Source: CAD feature listing. Evaluate the final solid. Frame: model axes, mm. A direction names the side the tool comes from. Give positions to 0.01 mm unless a question says otherwise; leave off trailing zeros. Loops run counter-clockwise (first coordinate to the right, second up) from the corner with the lowest first, then second, coordinate; pieces in that order, holes last.
from build123d import *

# Parameters (mm, degrees)
F0_W      = 79
F0_H      = 58
F0_W_2    = 69
F0_H_2    = 46
F1_DEPTH  = 2
F2_W      = 15
F2_H      = 5
F3_DEPTH  = 10
F5_DEPTH  = 20
F6_W      = 75
F6_H      = 20
F7_DEPTH  = 5
F8_R      = 1
F9_DEPTH  = 5
F10_R     = 1
F11_DEPTH = 79.001
F12_W     = 5
F12_H     = 2
F13_DEPTH = 69
F14_ANGLE = 180


with BuildPart() as f1:
    # F0 (on Top) → F1 (new body)
    with BuildSketch(Plane.XY):
        with Locations((-4.5810023546, -13.9063113923)):
            Rectangle(F0_W, F0_H)
        with Locations((-4.5810023546, -12.9063113923)):
            Rectangle(F0_W_2, F0_H_2, mode=Mode.SUBTRACT)
    extrude(amount=F1_DEPTH)

    # F2 (on face) → F3 (join)
    with BuildSketch(Plane(origin=(0, 0, 0), x_dir=(1, 0, 0), z_dir=(0, 0, -1))):
        with Locations((5.4189976454, -12.5936886077)):
            Rectangle(F2_W, F2_H)
        with Locations((-14.5810023546, -12.5936886077)):
            Rectangle(F2_W, F2_H)
    extrude(amount=F3_DEPTH)

    # F4 (on face) → F5 (join)
    with BuildSketch(Plane(origin=(0, 0, 0), x_dir=(1, 0, 0), z_dir=(0, 0, -1))):
        Polygon((34.9189976454, 35.9063113923), (34.9189976454, 42.9063113923), (-44.0810023546, 42.9063113923), (-44.0810023546, 35.9063113923), (-39.0810023546, 35.9063113923), (29.9189976454, 35.9063113923), align=None)
    extrude(amount=F5_DEPTH)

    # F6 (on face) → F7 (cut)
    with BuildSketch(Plane.XZ.offset(42.9063113923)):
        with Locations((-4.5810023546, -10)):
            Rectangle(F6_W, F6_H)
    extrude(amount=-F7_DEPTH, mode=Mode.SUBTRACT)

    # F8 (on face) → F9 (cut, through all)
    with BuildSketch(Plane(origin=(0, 15.0936886077, 0), x_dir=(-1, 0, 0), z_dir=(0, 1, 0))):
        with Locations((-5.4189976454, -5)):
            Circle(F8_R)
        with Locations((14.5810023546, -5)):
            Circle(F8_R)
    extrude(amount=-F9_DEPTH, mode=Mode.SUBTRACT)

    # F10 (on face) → F11 (cut, through all)
    with BuildSketch(Plane(origin=(-44.0810023546, 0, 0), x_dir=(0, -1, 0), z_dir=(-1, 0, 0))):
        with Locations((39.4063113923, -10)):
            Circle(F10_R)
    extrude(amount=-F11_DEPTH, mode=Mode.SUBTRACT)

    # F12 (on face) → F13 (join, through all)
    with BuildSketch(Plane(origin=(29.9189976454, 0, 0), x_dir=(0, -1, 0), z_dir=(-1, 0, 0))):
        with Locations((13.4063113923, 1)):
            Rectangle(F12_W, F12_H)
    extrude(amount=F13_DEPTH)


with BuildPart() as f1_1:
    # F14: moved
    add(f1.part.rotate(Axis((-4.5810023546, -10.9063113923, 2), (1, 0, 0)), F14_ANGLE))


solid = f1_1.part
1) Reachability of faces 1 (the flat face through (-15, -34, 14)), 2 (the cylindrical face through (6.156, -34.441, 8.324)), 3 (the flat face through (29.919, -21, 3)) from +Z, -Z, +X, -X, +Y, -Y: full face, straight path, thin tool, end or side. Return the list, or none.
Checks:
face 1: +Z, +X, -X, -Y
face 2: -Y
face 3: +Z, -Z
2) Contact query for flat-ended pins moving along their axis: P1, Ø5.5, axis at x = -12, y = -33.5, coming from the +Z side; P2, Ø1.5, axis at y = -35, z = 6.5, coming from the -X side; P3, Ø12, axis at x = -9, z = 22, coming from the -Y side; P4, Ø2, axis at y = 8.5, z = 6.5, coming from the -X side. Output: stop coordinate, or through.
Checks:
P1: stops at z = 14
P2: stops at x = -22.08
P3: stops at y = 14.09
P4: passes through
3) Cut plane A-A (z = 9). Return loops of the section in (x, y), and give its area (3 significant figures).
Checks:
outline: (-44.08, 14.09) - (34.92, 14.09) - (34.92, 21.09) - (32.92, 21.09) - (32.92, 16.09) - (-42.08, 16.09) - (-42.08, 21.09) - (-44.08, 21.09) - close; (-22.08, -36.91) - (-15.58, -36.91) - (-15.58, -31.91) - (-22.08, -31.91) - close; (-13.58, -36.91) - (-7.08, -36.91) - (-7.08, -31.91) - (-13.58, -31.91) - close; (-2.08, -36.91) - (4.42, -36.91) - (4.42, -31.91) - (-2.08, -31.91) - close; (6.42, -36.91) - (12.92, -36.91) - (12.92, -31.91) - (6.42, -31.91) - close
area: 308 mm2
4) Cut plane C-C (x = 25.5). Return loops of the section in (y, z).
Checks:
outline: (-36.91, 2) - (-31.91, 2) - (-31.91, 4) - (-36.91, 4) - close; (-10.91, 2) - (-5.91, 2) - (-5.91, 4) - (-10.91, 4) - close; (14.09, 2) - (21.09, 2) - (21.09, 4) - (16.09, 4) - (16.09, 24) - (14.09, 24) - close
5) Pull-direction query (Y, two-part tool) for faces 4 (the flat face through (29.919, 4, 3)), 5 (the flat face through (4, -36.906, 7)), 6 (the cylindrical face through (33.905, 17.377, 14.976)), 7 (the flat face through (-5, 19, 4)); classes: released by +Y, released by -Y, zero draft, split by the parting line, or undercut.
Checks:
face 4: undercut
face 5: released by -Y
face 6: undercut
face 7: zero draft
6) Ray query, probe 1 along Y at (x, z) = (-24, 3.75); probe 2 along Y at (x, z) = (-42.9, 14); probe 3 along Y at (x, z) = (-33.5, 7.75). Return the intervals inside material, ascending.
Checks:
probe 1: y = -36.91 to -31.91, -10.91 to -5.91, 14.09 to 21.09
probe 2: y = 14.09 to 16.59, 18.59 to 21.09
probe 3: y = 14.09 to 16.09
7) Cut plane D-D (z = 22.5). Return loops of the section in (x, y), and give its area (3 significant figures).
Checks:
outline: (-44.08, 14.09) - (34.92, 14.09) - (34.92, 21.09) - (32.92, 21.09) - (32.92, 16.09) - (-42.08, 16.09) - (-42.08, 21.09) - (-44.08, 21.09) - close
area: 178 mm2
8) Cut plane B-B (y = -23). Return loops of the section in (x, z).
Checks:
outline: (-44.08, 2) - (-39.08, 2) - (-39.08, 4) - (-44.08, 4) - close; (29.92, 2) - (34.92, 2) - (34.92, 4) - (29.92, 4) - close
